Source: CAD feature listing. Evaluate the final solid. Frame: model axes, mm. A direction names the side the tool comes from. Coordinates: 2 decimals unless noted, no trailing zeros. Loops run counter-clockwise (first coordinate to the right, second up) from the corner with the lowest first, then second, coordinate; pieces in that order, holes last.
Item 1: Section query D-D, the plane y = 32. Return the cut outline in (x, z), then the cut area to 3 significant figures.
Item 2: Section query A-A, the plane y = 0. Return the cut outline in (x, z), then the cut area to 3 significant figures.
Item 3: Line query: probe 1 along X at (y, z) = (-36.75, 9.9); probe 2 along Z at (x, y) = (-0.5, 37); probe 3 along X at (y, z) = (1, 19). Output: solid intervals per line, ascending.
Item 4: Pin query (flat end, axial travel): pin 1 Ø1.2 at (x, y) = (18.5, -37.5) entering from +Z; pin 2 Ø1.2 at (x, z) = (-13.5, 18.5) entering from +Y; pin 3 Ø0.8 at (y, z) = (-24.5, 16.5) entering from +X; pin 4 Ø12 at (y, z) = (-33, 20.5) entering from +X. Return the tip coordinate at first contact, or that it passes through.
Item 5: Section query C-C, the plane z = -5. Return the cut outline in (x, y), then the cut area to 3 significant figures.
Item 6: Section query B-B, the plane x = -4. Return the cut outline in (y, z), then the cut area to 3 significant figures.
Item 7: Pull-direction query (X, two-part tool) for faces 4 (the flat face through (27.5, 0, 14)), 5 (the flat face through (-4, 0, 4)), 6 (the flat face through (0, -12, 0)); classes: +X half, -X half, draft (parallel to the pull), parting line (faces both ways), or undercut.
Item 8: Reachability of faces 1 (the cylindrical face through (2.395, -10.787, 0.986)), 2 (the flat face through (0, 55.5, 39)), 3 (the cylindrical face through (24.9, 19.7, 19.9)) from +Z, -Z, +X, -X, +Y, -Y: full face, straight path, thin tool, end or side. Return the list, or none.
```python
from build123d import *

# Parameters (mm, degrees)
CROQUIS4_R                  = 2.5
SALIENTE_EXTRUIR1_DEPTH     = 4
CROQUIS5_R                  = 20
SALIENTE_EXTRUIR2_DEPTH     = 8.5
SALIENTE_EXTRUIR4_START     = -3
SALIENTE_EXTRUIR4_DEPTH     = 3
REDONDEO1_R                 = 10
SALIENTE_EXTRUIR5_OUTLINE_R = 2
SALIENTE_EXTRUIR5_DEPTH     = 15
CROQUIS9_R                  = 1.6
CORTAR_EXTRUIR1_DEPTH       = 70.417217007
CROQUIS11_W                 = 35
CROQUIS11_H                 = 50
SALIENTE_EXTRUIR7_DEPTH     = 7
CROQUIS12_W                 = 35
CROQUIS12_H                 = 7
SALIENTE_EXTRUIR8_DEPTH     = 28
CHAFL_N2_SIZE               = 7
CROQUIS13_R                 = 11.05
CORTAR_EXTRUIR2_DEPTH       = 2


# Read off the part's stored shape, not the designer's step: Saliente-Extruir5
with BuildPart() as part:
    # Croquis4 → Saliente-Extruir1 (new body)
    with BuildSketch(Plane.XY):
        with BuildLine():
            Line((-17.5, 27.5), (17.5, 27.5))
            ThreePointArc((17.5, 27.5), (24.571067812, 24.571067812), (27.5, 17.5))
            Line((27.5, 17.5), (27.5, -17.5))
            ThreePointArc((27.5, -17.5), (24.571067812, -24.571067812), (17.5, -27.5))
            Line((17.5, -27.5), (-17.5, -27.5))
            ThreePointArc((-17.5, -27.5), (-24.571067812, -24.571067812), (-27.5, -17.5))
            Line((-27.5, -17.5), (-27.5, 17.5))
            ThreePointArc((-27.5, 17.5), (-24.571067812, 24.571067812), (-17.5, 27.5))
        make_face()
        Circle(CROQUIS4_R, mode=Mode.SUBTRACT)
    extrude(amount=SALIENTE_EXTRUIR1_DEPTH)

    # Croquis5 → Saliente-Extruir2 (add)
    with BuildSketch(Plane.XY.offset(4)):
        with BuildLine():
            Line((-17.5, 27.5), (17.5, 27.5))
            ThreePointArc((17.5, 27.5), (24.571067812, 24.571067812), (27.5, 17.5))
            Line((27.5, 17.5), (27.5, -17.5))
            ThreePointArc((27.5, -17.5), (24.571067812, -24.571067812), (17.5, -27.5))
            Line((17.5, -27.5), (-17.5, -27.5))
            ThreePointArc((-17.5, -27.5), (-24.571067812, -24.571067812), (-27.5, -17.5))
            Line((-27.5, -17.5), (-27.5, 17.5))
            ThreePointArc((-27.5, 17.5), (-24.571067812, 24.571067812), (-17.5, 27.5))
        make_face()
        Circle(CROQUIS5_R, mode=Mode.SUBTRACT)
    extrude(amount=SALIENTE_EXTRUIR2_DEPTH)

    # Croquis6 → Saliente-Extruir4 (add)
    with BuildSketch(Plane.XY.offset(12.5).offset(SALIENTE_EXTRUIR4_START)):
        with BuildLine():
            Line((-25.720640569, -23.193950178), (-15, -57.5))
            Line((-15, -57.5), (15, -57.5))
            Line((15, -57.5), (25.720640569, -23.193950178))
            ThreePointArc((25.720640569, -23.193950178), (22.140069947, -26.358315353), (17.5, -27.5))
            Line((17.5, -27.5), (-17.5, -27.5))
            ThreePointArc((-17.5, -27.5), (-22.140069947, -26.358315353), (-25.720640569, -23.193950178))
        make_face()
    extrude(amount=SALIENTE_EXTRUIR4_DEPTH)

    # Redondeo1
    # the kernel refuses this fillet: 10 mm, written as the material it adds along each edge
    with BuildSketch(Plane(origin=(17.5, -17.5, 9.5), x_dir=(-0.31521717271258337, 0.949019564617656, 0), z_dir=(-0.949019564617656, -0.31521717271258337, 0))) as redondeo1_piece_1_section:
        with BuildLine():
            CenterArc((19.987492178, 10), REDONDEO1_R, 182.865983983, 87.134016017)
            Line((19.987492178, 0), (10, 0))
            Line((10, 0), (10, 9.5))
        make_face()
    redondeo1_piece_1 = revolve(axis=Axis((17.5, -17.5, 9.5), (0, 0, -1)), revolution_arc=198.373924806, mode=Mode.PRIVATE)
    redondeo1_piece_1 = split(redondeo1_piece_1, bisect_by=Plane(origin=(27.5, -26.624186886, 2.060383814), z_dir=(-1, 0, 0)), keep=Keep.TOP, mode=Mode.PRIVATE)
    redondeo1_piece_1 = redondeo1_piece_1 - Plane(origin=(0, 0, 2.060383814), x_dir=(1, 0, 0), z_dir=(0, 0, -1)) * Cylinder(20, 80, mode=Mode.PRIVATE)
    redondeo1_piece_1 = split(redondeo1_piece_1, bisect_by=Plane(origin=(24.437894836, -27.298736526, 2.060383814), z_dir=(-0.9544799780350299, 0.2982749931359464, 0)), keep=Keep.TOP, mode=Mode.PRIVATE)
    add(redondeo1_piece_1)
    with BuildSketch(Plane(origin=(-17.5, -17.5, 9.5), x_dir=(0, -1, 0), z_dir=(1, 0, 0))) as redondeo1_piece_2_section:
        with BuildLine():
            CenterArc((19.987492178, 10), REDONDEO1_R, 182.865983983, 87.134016017)
            Line((19.987492178, 0), (10, 0))
            Line((10, 0), (10, 9.5))
        make_face()
    redondeo1_piece_2 = revolve(axis=Axis((-17.5, -17.5, 9.5), (0, 0, -1)), revolution_arc=198.373924806, mode=Mode.PRIVATE)
    redondeo1_piece_2 = split(redondeo1_piece_2, bisect_by=Plane(origin=(-27.5, -26.624186886, 2.060383814), z_dir=(1, 0, 0)), keep=Keep.TOP, mode=Mode.PRIVATE)
    redondeo1_piece_2 = redondeo1_piece_2 - Plane(origin=(0, 0, 2.060383814), x_dir=(1, 0, 0), z_dir=(0, 0, -1)) * Cylinder(20, 80, mode=Mode.PRIVATE)
    redondeo1_piece_2 = split(redondeo1_piece_2, bisect_by=Plane(origin=(-24.437894836, -27.298736526, 2.060383814), z_dir=(0.9544799780350299, 0.29827499313594635, 0)), keep=Keep.TOP, mode=Mode.PRIVATE)
    add(redondeo1_piece_2)
    with BuildSketch(Plane(origin=(17.5, -27.5, 9.5), x_dir=(0, 0, -1), z_dir=(-1, 0, 0))) as redondeo1_piece_3:
        with BuildLine():
            CenterArc((10, 9.987492178), REDONDEO1_R, 180, 87.134016017)
            Line((0, 9.987492178), (0, 0))
            Line((0, 0), (9.5, 0))
        make_face()
    extrude(amount=35)

    # Saliente-Extruir5 outline → Saliente-Extruir5 (add)
    with BuildSketch(Plane.XY.offset(12.5)):
        with BuildLine():
            ThreePointArc((-27.5, -17.5), (-27.04479978, -20.482749931), (-25.720640569, -23.193950178))
            Line((-25.720640569, -23.193950178), (-15, -57.5))
            Line((-15, -57.5), (-12.5, -57.5))
            Line((-12.5, -57.5), (-12.5, -55.5))
            Line((-12.5, -55.5), (-15, -55.5))
            Line((-15, -55.5), (-15, -25))
            Line((-15, -25), (-11.560632513, -25))
            Line((-11.560632513, -25), (-11.560632513, -24.25))
            Line((-11.560632513, -24.25), (-22.25, -24.25))
            ThreePointArc((-22.25, -24.25), (-25.19427191, -20.722135955), (-26.25, -16.25))
            Line((-26.25, -16.25), (-26.25, 16.25))
            ThreePointArc((-26.25, 16.25), (-26.205571214, 17.191595354), (-26.072679638, 18.12482392))
            ThreePointArc((-26.072679638, 18.12482392), (-24.934779512, 19.680078923), (-23.010409798, 19.782235789))
            ThreePointArc((-23.010409798, 19.782235789), (-20.782444846, 20.273260806), (-20.464111601, 22.532375088))
            ThreePointArc((-20.464111601, 22.532375088), (-20.519074057, 24.539569231), (-19.008189542, 25.862096049))
            ThreePointArc((-19.008189542, 25.862096049), (-17.64266642, 26.152549179), (-16.25, 26.25))
            Line((-16.25, 26.25), (16.25, 26.25))
            ThreePointArc((16.25, 26.25), (17.64266642, 26.152549179), (19.008189542, 25.862096049))
            ThreePointArc((19.008189542, 25.862096049), (20.519074057, 24.539569231), (20.464111601, 22.532375088))
            ThreePointArc((20.464111601, 22.532375088), (20.782444846, 20.273260806), (23.010409798, 19.782235789))
            ThreePointArc((23.010409798, 19.782235789), (24.934779512, 19.680078923), (26.072679638, 18.12482392))
            ThreePointArc((26.072679638, 18.12482392), (26.205571214, 17.191595354), (26.25, 16.25))
            Line((26.25, 16.25), (26.25, -16.25))
            ThreePointArc((26.25, -16.25), (25.19427191, -20.722135955), (22.25, -24.25))
            Line((22.25, -24.25), (11.560632513, -24.25))
            Line((11.560632513, -24.25), (11.560632513, -25))
            Line((11.560632513, -25), (15, -25))
            Line((15, -25), (15, -55.5))
            Line((15, -55.5), (12.5, -55.5))
            Line((12.5, -55.5), (12.5, -57.5))
            Line((12.5, -57.5), (15, -57.5))
            Line((15, -57.5), (25.720640569, -23.193950178))
            ThreePointArc((25.720640569, -23.193950178), (27.04479978, -20.482749931), (27.5, -17.5))
            Line((27.5, -17.5), (27.5, 17.5))
            ThreePointArc((27.5, 17.5), (24.571067812, 24.571067812), (17.5, 27.5))
            Line((17.5, 27.5), (-17.5, 27.5))
            ThreePointArc((-17.5, 27.5), (-24.571067812, 24.571067812), (-27.5, 17.5))
            Line((-27.5, 17.5), (-27.5, -17.5))
        make_face()
        with Locations((-18, -36.75)):
            Circle(SALIENTE_EXTRUIR5_OUTLINE_R, mode=Mode.SUBTRACT)
        with Locations((18, -36.75)):
            Circle(SALIENTE_EXTRUIR5_OUTLINE_R, mode=Mode.SUBTRACT)
    extrude(amount=SALIENTE_EXTRUIR5_DEPTH)

    # Croquis9 → Cortar-Extruir1 (cut, through all)
    with BuildSketch(Plane.XY.offset(27.5)):
        with Locations((-22.25, 21.632040357)):
            Circle(CROQUIS9_R)
        with Locations((-18, -36.75)):
            Circle(CROQUIS9_R)
        with Locations((18, -36.75)):
            Circle(CROQUIS9_R)
        with Locations((22.25, 21.632040357)):
            Circle(CROQUIS9_R)
    extrude(amount=-CORTAR_EXTRUIR1_DEPTH, mode=Mode.SUBTRACT)

    # Croquis11 → Saliente-Extruir7 (add)
    with BuildSketch(Plane(origin=(0, 27.5, 0), x_dir=(1, 0, 0), z_dir=(0, 1, 0))):
        with Locations((0, -10)):
            Rectangle(CROQUIS11_W, CROQUIS11_H)
    extrude(amount=SALIENTE_EXTRUIR7_DEPTH)

    # Croquis12 → Saliente-Extruir8 (add)
    with BuildSketch(Plane.XZ.offset(-27.5)):
        with Locations((0, 38.5)):
            Rectangle(CROQUIS12_W, CROQUIS12_H)
        with Locations((0, -18.5)):
            Rectangle(CROQUIS12_W, CROQUIS12_H)
    extrude(amount=-SALIENTE_EXTRUIR8_DEPTH)

    # Chaflán2
    chafl_n2_edges = [part.edges().sort_by_distance(p)[0] for p in [
        (0, 27.5, 0),
    ]]
    chamfer(chafl_n2_edges, length=CHAFL_N2_SIZE)

    # Croquis13 → Cortar-Extruir2 (cut)
    with BuildSketch(Plane(origin=(0, 0, 0), x_dir=(-1, 0, 0), z_dir=(0, 0, -1))):
        Circle(CROQUIS13_R)
    extrude(amount=-CORTAR_EXTRUIR2_DEPTH, mode=Mode.SUBTRACT)


solid = part.part
```
Verdict:
1. outline: (-17.5, -22) - (17.5, -22) - (17.5, 42) - (-17.5, 42) - close
1. area: 2,240 mm2
2. outline: (-27.5, 0) - (-11.05, 0) - (-11.05, 2) - (-2.5, 2) - (-2.5, 4) - (-20, 4) - (-20, 12.5) - (-26.25, 12.5) - (-26.25, 27.5) - (-27.5, 27.5) - close; (2.5, 2) - (11.05, 2) - (11.05, 0) - (27.5, 0) - (27.5, 27.5) - (26.25, 27.5) - (26.25, 12.5) - (20, 12.5) - (20, 4) - (2.5, 4) - close
2. area: 331 mm2
3. probe 1: x = -21.48 to -19.6, -16.4 to 16.4, 19.6 to 21.48
3. probe 2: z = -22 to -15, 35 to 42
3. probe 3: x = -27.5 to -26.25, 26.25 to 27.5
4. pin 1: passes through
4. pin 2: stops at y = 34.5
4. pin 3: stops at x = 25.44
4. pin 4: stops at x = 24.53
5. outline: (-17.5, 25.5) - (17.5, 25.5) - (17.5, 34.5) - (-17.5, 34.5) - close
5. area: 315 mm2
6. outline: (-57.5, 9.5) - (-37.49, 9.5) arc R10 cw to (-27.5, 0) - (-10.3, 0) - (-10.3, 2) - (10.3, 2) - (10.3, 0) - (20.5, 0) - (27.5, -7) - (27.5, -22) - (55.5, -22) - (55.5, -15) - (34.5, -15) - (34.5, 35) - (55.5, 35) - (55.5, 42) - (27.5, 42) - (27.5, 27.5) - (26.25, 27.5) - (26.25, 12.5) - (19.6, 12.5) - (19.6, 4) - (-19.6, 4) - (-19.6, 12.5) - (-57.5, 12.5) - close
6. area: 1,210 mm2
7. face 4: +X half
7. face 5: undercut
7. face 6: draft
8. face 1: -Z
8. face 2: +Z, -Z, +X, -X, +Y
8. face 3: +Z
